Geometry check sheet. Reference: the model listing, model coordinates, mm. Face numbers are marked on the shaded views. A direction names the side the tool comes from. Coordinates: 2 decimals unless noted, no trailing zeros. Write each loop counter-clockwise with the first axis right and the second up, starting at its lowest first coordinate (ties: lowest second). Pieces come first, ordered by that corner, then holes. Notation, with made-up numbers: (30, -20) -> (87, -20) arc R21 ccw to (87, -5) -> close; hole circle Ø11 at (-1.5, -28). An arc over 180 degrees is marked (long way). Answer in a Markdown table with one row per item. Add a question column.
Q1. Section check A-A, the plane x = 0. Record the boundary of the cut face in (y, z).
Q2. Thickness scan on line 1 (Z direction, x = -3.5, y = -0.5); line 2 (Z direction, x = 4.5, y = 3.25); line 3 (Z direction, x = 0, y = -2.75). Record the ranges inside material, lowest first.
Q3. Tool access check on the marked faces 1 and 2. Record the directions out of +Z, -Z, +X, -X, +Y, -Y that give a thin tool (end or side, any length) a straight path to the whole face; none if there is none.
Q4. Section check D-D, the plane z = -16.5. Record the boundary of the cut face in (x, y), and give its area (3 significant figures).
Q5. Gauge pin test, flat ends, axial feed: P1, Ø5, axis at x = 0.5, z = -13, coming from the +Y side; P2, Ø1.5, axis at y = -3.5, z = -10.5, coming from the -X side; P3, Ø1.5, axis at x = -6, z = -11, coming from the -Y side; P4, Ø1.5, axis at x = -6, y = 5, coming from the -Z side. Record the tip position at first contact, or that the pin passes through.
Q6. Section check C-C, the plane z = -9. Record the boundary of the cut face in (x, y).
```python
from build123d import *

# Parameters (mm, degrees)
SKETCH1_W     = 5.5
SKETCH1_H     = 8
CHAMFER1_SIZE = 0.5
CHAMFER2_SIZE = 0.5


with BuildPart() as part:
    # Sketch1 → Revolve1 (revolve)
    with BuildSketch(Plane(origin=(0, 0, 0), x_dir=(0, 0, -1), z_dir=(1, 0, 0)), mode=Mode.PRIVATE) as revolve1_sk:
        with Locations((2.75, 4)):
            Rectangle(SKETCH1_W, SKETCH1_H)
        with BuildLine():
            Line((5.5, 4), (5.5, 0))
            Line((5.5, 0), (20, 0))
            Line((20, 0), (20, 4))
            Line((20, 4), (17, 4))
            ThreePointArc((17, 4), (15.5, 2.5), (14, 4))
            Line((14, 4), (5.5, 4))
        make_face()
    revolve(revolve1_sk.sketch.rotate(Axis((0, 0, -5.5), (0, 0, -1)), 90), axis=Axis((0, 0, -5.5), (0, 0, -1)))

    # Chamfer1
    chamfer1_edges = [part.edges().sort_by_distance(p)[0] for p in [
        (-8, 0, 0),
    ]]
    chamfer(chamfer1_edges, length=CHAMFER1_SIZE)

    # Chamfer2
    chamfer2_edges = [part.edges().sort_by_distance(p)[0] for p in [
        (-4, 0, -20),
    ]]
    chamfer(chamfer2_edges, length=CHAMFER2_SIZE)


solid = part.part
```
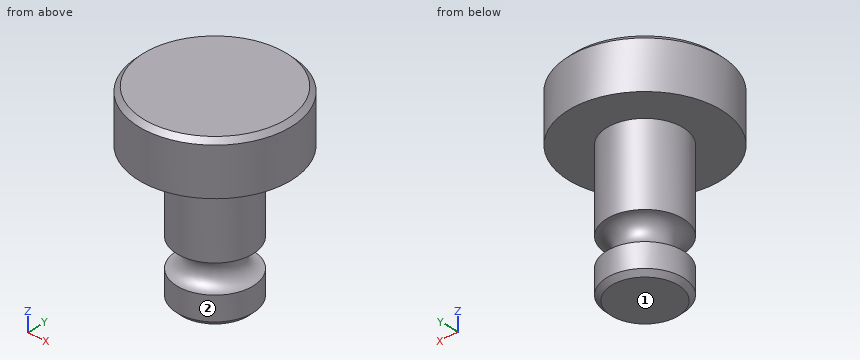
Calculated:
| question | item | result |
|---|---|---|
| 1 | outline | (-8, -5.5) -> (-4, -5.5) -> (-4, -14) arc R1.5 cw to (-4, -17) -> (-4, -19.5) -> (-3.5, -20) -> (3.5, -20) -> (4, -19.5) -> (4, -17) arc R1.5 cw to (4, -14) -> (4, -5.5) -> (8, -5.5) -> (8, -0.5) -> (7.5, 0) -> (-7.5, 0) -> (-8, -0.5) -> close |
| 2 | line 1 | z = -19.96 to -16.93, -14.07 to 0 |
| 2 | line 2 | z = -5.5 to 0 |
| 2 | line 3 | z = -20 to -16.33, -14.67 to 0 |
| 3 | face 1 | -Z, +X, -X, +Y, -Y |
| 3 | face 2 | -Z |
| 4 | outline | circle Ø5.76 at (0, 0) |
| 4 | area | 26.1 mm² |
| 5 | P1 | stops at y = 4 |
| 5 | P2 | stops at x = -2.9 |
| 5 | P3 | passes through |
| 5 | P4 | stops at z = -5.5 |
| 6 | outline | circle Ø8 at (0, 0) |
